Print and shaded views of the part. All mm, measured from the part's lowest x, y and z. A direction names the side the tool comes from. Round coordinates to 2 decimals unless told otherwise and drop trailing zeros. Write each loop counter-clockwise with the first axis right and the second up, starting at its lowest first coordinate (ties: lowest second). Pieces come first, ordered by that corner, then holes. Notation, with made-up numbers: M 76,-3.5 L 97,-3.5 A26 cw 97,32.5 Z; hole C -4.5,41.25 d5. An arc over 180 degrees is marked long. Write item = value, one per line.
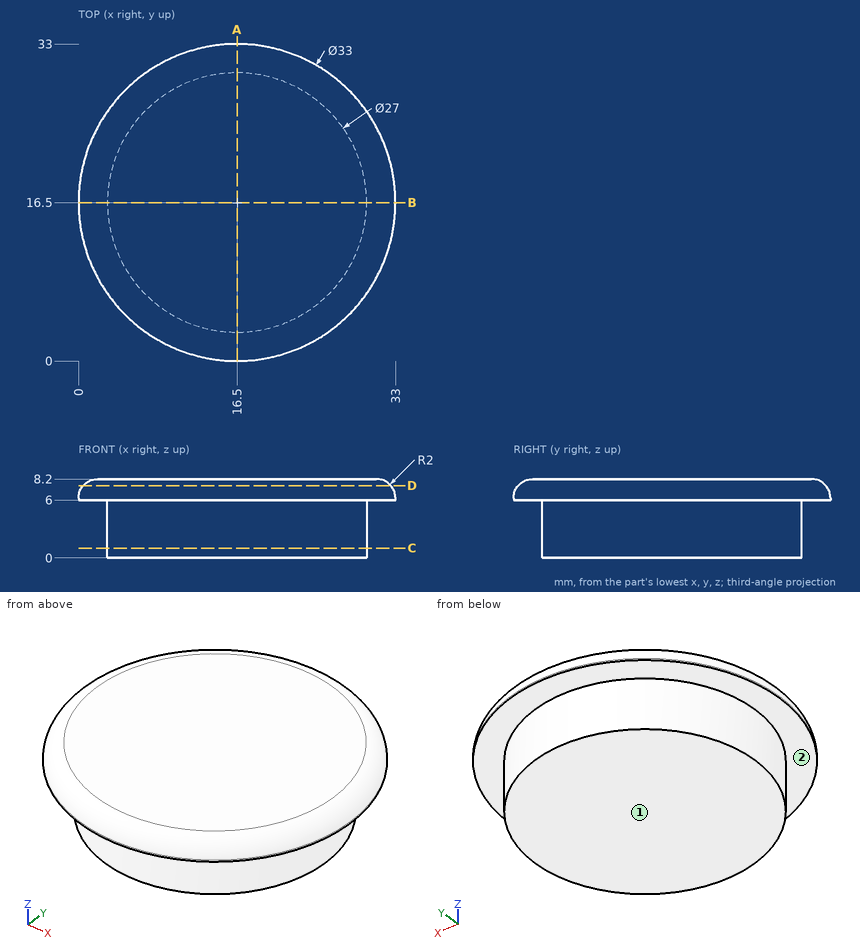
1. Band-saw the part on A-A (x = 16.5). List the corners of the cut face in (y, z), plus the area to 3 significant figures.
Responses:
outline = M 0,6 L 3,6 L 3,0 L 30,0 L 30,6 L 33,6 L 33,6.2 A2 ccw 31,8.2 L 2,8.2 A2 ccw 0,6.2 Z
area = 233 mm²
2. Probe probe 1 along X at (y, z) = (17, 6.25); probe 2 along Z at (x, y) = (17.5, 30.5); probe 3 along Y at (x, z) = (17, 5). List the from-to ranges inside material, lowest first.
Responses:
probe_1 = 0.01 to 32.99
probe_2 = 6 to 8.2
probe_3 = 3.01 to 29.99
3. Tool access for the marked faces 1 and 2: list every direction of +Z, -Z, +X, -X, +Y, -Y with a clear straight run to the whole face (end or side of a thin tool).
Responses:
face_1 = -Z, +X, -X, +Y, -Y
face_2 = -Z
4. Flat gauge pins, fed straight in: pin 1 (1.5 mm diameter, centred on y = 23, z = 1.5, fed in from +X); pin 2 (4 mm diameter, centred on y = 6.5, z = 6, fed in from -X); pin 3 (1 mm diameter, centred on x = 23, z = 5, fed in from +Y); pin 4 (10 mm diameter, centred on x = 22, y = 13.5, fed in from -Z). Where does each tip first touch, or does it go through?
Responses:
pin_1 = 28.71
pin_2 = 2.07
pin_3 = 28.59
pin_4 = 0
5. Band-saw the part on C-C (z = 1). List the corners of the cut face in (x, y).
Responses:
outline = C 16.5,16.5 d27
6. Band-saw the part on D-D (z = 7.5). List the corners of the cut face in (x, y), plus the area to 3 significant figures.
Responses:
outline = C 16.5,16.5 d32.04
area = 806 mm²
